from build123d import *

# Parameters (mm, degrees)
SKETCH1_W       = 203.2
SKETCH1_H       = 76.2
PLATE_DEPTH     = 9.525
SKETCH2_R       = 3.175
SEED_HOLE_DEPTH = 218.226622735


with BuildPart() as part:
    # Sketch1 → plate (new body)
    with BuildSketch(Plane.XY):
        with Locations((101.6, 38.1)):
            Rectangle(SKETCH1_W, SKETCH1_H)
    extrude(amount=PLATE_DEPTH)

    # Sketch2 → seed_hole (cut, through all)
    with BuildSketch(Plane.XY):
        with Locations((25.4, 38.1)):
            Circle(SKETCH2_R)
    extrude(amount=SEED_HOLE_DEPTH, mode=Mode.SUBTRACT)


solid = part.part
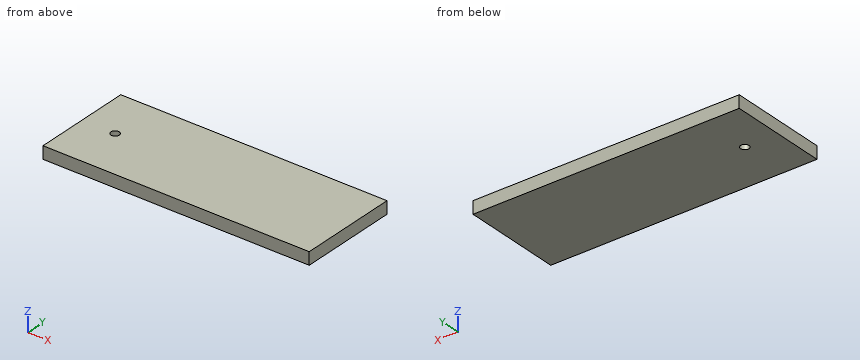
Could you check a few things on this model? Use its own coordinates, in mm. Give positions to 0.01 mm unless a question says otherwise; leave off trailing zeros. Loops run counter-clockwise (first coordinate to the right, second up) from the corner with the lowest first, then second, coordinate; pieces in that order, holes last. Notation, with made-up numbers: (34.5, 24.5) -> (91.5, 24.5) arc R19 ccw to (91.5, 49.5) -> close; hole circle Ø10 at (34, 85.25). An arc over 180 degrees is marked (long way). Return JSON: item names as keys, results as strings.
Item 1: If we section it at A-A on x = 25.4: List the corners of the cut face in (y, z) for me (3 decimals), plus the area to 3 significant figures.
Geometry results:
{"outline": "(0, 0) -> (34.925, 0) -> (34.925, 9.525) -> (0, 9.525) -> close; (41.275, 0) -> (76.2, 0) -> (76.2, 9.525) -> (41.275, 9.525) -> close", "area": "665 mm²"}
Item 2: I need wall thicknesses on L1, parallel to X at y = 38.1, z = 3 (3 decimals); L2, parallel to Y at x = 25.4, z = 4.25 (3 decimals). Which ranges of each line are inside material? Lowest first, please. Write a range as from..to.
Geometry results:
{"L1": "x = 0..22.225, 28.575..203.2", "L2": "y = 0..34.925, 41.275..76.2"}
Item 3: I'm going to push a flat-ended pin straight in: pin 1 (4 mm diameter, centred on x = 25.4, y = 38.1, fed in from +Z). Where does the tip first touch, or does it pass through?
Geometry results:
{"pin 1": "passes through"}
Item 4: If we section it at B-B on y = 38.1: List the corners of the cut face in (x, z) for me (3 decimals), plus the area to 4 significant figures.
Geometry results:
{"outline": "(0, 0) -> (22.225, 0) -> (22.225, 9.525) -> (0, 9.525) -> close; (28.575, 0) -> (203.2, 0) -> (203.2, 9.525) -> (28.575, 9.525) -> close", "area": "1,875 mm²"}
